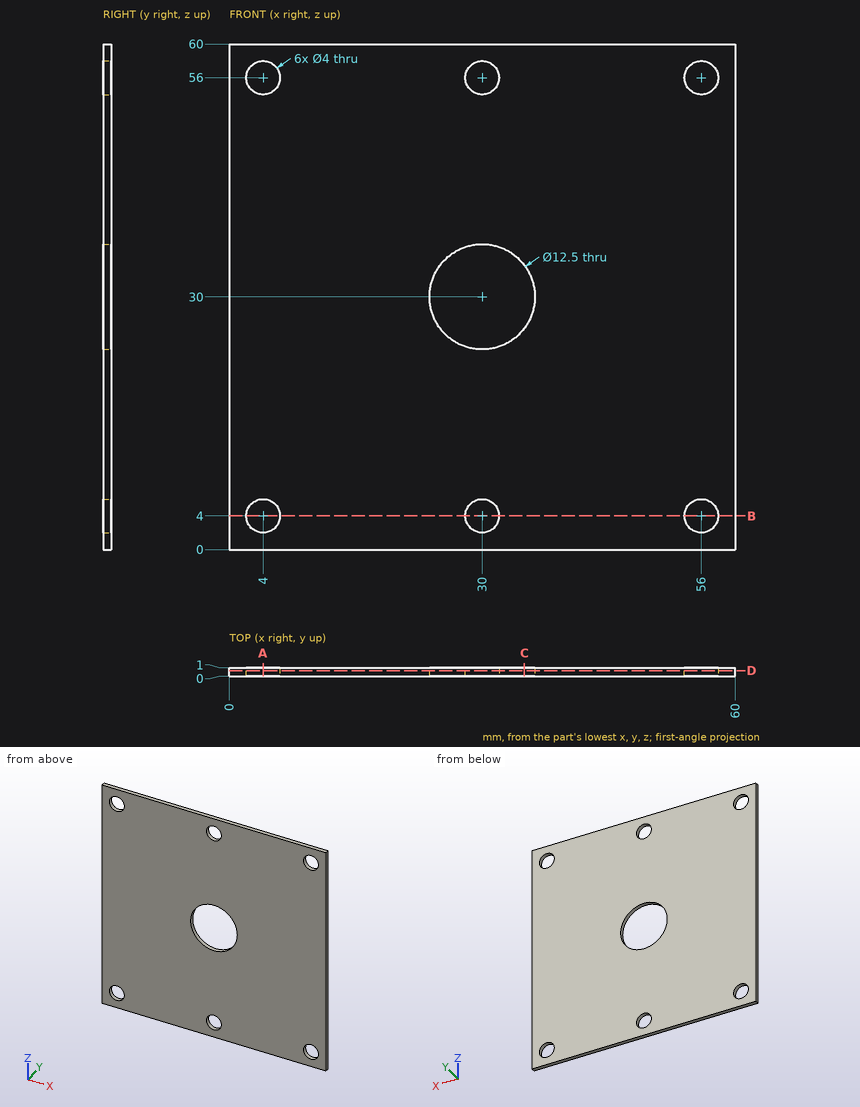
Part print with two shaded views. Sizes in mm from the minimum x, y, z corner. Round coordinates to 2 decimals unless told otherwise and drop trailing zeros. Order: outer loops, then holes, each group sorted by start corner. A loop starts at its lowest first (then second) coordinate and runs counter-clockwise, first axis right, second up.
(1) Band-saw the part on B-B (z = 4). List the corners of the cut face in (x, y), then the cut area to 3 significant figures.
(2) Pin check, flat tip, straight feed: pin 1 (2.5 mm diameter, centred on x = 30, z = 56, fed in from +Y). Stop position of the tip, or through.
(3) Band-saw the part on A-A (x = 4). List the corners of the cut face in (y, z).
(4) Band-saw the part on D-D (y = 0.65). List the corners of the cut face in (x, z), then the cut area to 3 significant figures.
(5) Drill centre lines: line 1 (Z direction, x = 30, y = 0.4); line 2 (X direction, y = 0.8, z = 4); line 3 (Z direction, x = 56, y = 0.5). Where is each one in solid material? Low to high.
(6) Band-saw the part on C-C (x = 35). List the corners of the cut face in (y, z).
Verdict:
1. outline: (0, 0) - (2, 0) - (2, 1) - (0, 1) - close; (6, 0) - (28, 0) - (28, 1) - (6, 1) - close; (32, 0) - (54, 0) - (54, 1) - (32, 1) - close; (58, 0) - (60, 0) - (60, 1) - (58, 1) - close
1. area: 48.0 mm2
2. pin 1: passes through
3. outline: (0, 0) - (1, 0) - (1, 2) - (0, 2) - close; (0, 6) - (1, 6) - (1, 54) - (0, 54) - close; (0, 58) - (1, 58) - (1, 60) - (0, 60) - close
4. outline: (0, 0) - (60, 0) - (60, 60) - (0, 60) - close; hole circle Ø4 at (4, 4); hole circle Ø4 at (4, 56); hole circle Ø12.5 at (30, 30); hole circle Ø4 at (30, 4); hole circle Ø4 at (30, 56); hole circle Ø4 at (56, 4); hole circle Ø4 at (56, 56)
4. area: 3,400 mm2
5. line 1: z = 0 to 2, 6 to 23.75, 36.25 to 54, 58 to 60
5. line 2: x = 0 to 2, 6 to 28, 32 to 54, 58 to 60
5. line 3: z = 0 to 2, 6 to 54, 58 to 60
6. outline: (0, 0) - (1, 0) - (1, 26.25) - (0, 26.25) - close; (0, 33.75) - (1, 33.75) - (1, 60) - (0, 60) - close
